```python
from build123d import *

# Parameters (mm, degrees)
SKETCH1_W                = 304.8
SKETCH1_H                = 304.8
BOSS_EXTRUDE1_DEPTH      = 2.54
SKETCH2_W                = 64.109804122
SKETCH2_H                = 40.213084064
BOSS_EXTRUDE2_DEPTH      = 31.75
BOSS_EXTRUDE2_TAPER      = 6
SKETCH3_R                = 6.35
CUT_EXTRUDE1_DEPTH       = 25.4
BOSS_EXTRUDE3_DEPTH      = 19.05
BOSS_EXTRUDE3_DEPTH_BACK = 19.05
SKETCH5_R                = 6.35
CUT_EXTRUDE2_DEPTH       = 50.8
SKETCH6_R                = 6.35
CUT_EXTRUDE3_DEPTH       = 19.05


with BuildPart() as part:
    # Sketch1 → Boss-Extrude1 (new body)
    with BuildSketch(Plane(origin=(0, 0, 0), x_dir=(1, 0, 0), z_dir=(0, 1, 0))):
        with Locations((152.4, 152.4)):
            Rectangle(SKETCH1_W, SKETCH1_H)
    extrude(amount=BOSS_EXTRUDE1_DEPTH)

    # Sketch2 → Boss-Extrude2 (add)
    with BuildSketch(Plane(origin=(0, 2.54, 0), x_dir=(1, 0, 0), z_dir=(0, 1, 0))):
        with Locations((152.4, 228.6)):
            Rectangle(SKETCH2_W, SKETCH2_H)
    extrude(amount=BOSS_EXTRUDE2_DEPTH, taper=BOSS_EXTRUDE2_TAPER)

    # Sketch3 → Cut-Extrude1 (cut)
    with BuildSketch(Plane(origin=(0, 34.29, 0), x_dir=(1, 0, 0), z_dir=(0, 1, 0))):
        with Locations((152.4, 228.6)):
            Circle(SKETCH3_R)
    extrude(amount=-CUT_EXTRUDE1_DEPTH, mode=Mode.SUBTRACT)

    # Sketch4 → Boss-Extrude3 (add, two sides)
    with BuildSketch(Plane(origin=(152.4, 0, 0), x_dir=(0, 0, -1), z_dir=(1, 0, 0))) as boss_extrude3_sk:
        Polygon((209.648741009, 34.29), (247.551258991, 34.29), (247.551258991, 36.83), (212.188741009, 36.83), (212.188741009, 77.47), (212.188741009, 85.09), (209.648741009, 85.09), align=None)
    extrude(amount=BOSS_EXTRUDE3_DEPTH)
    extrude(boss_extrude3_sk.sketch, amount=-BOSS_EXTRUDE3_DEPTH_BACK)

    # Sketch5 → Cut-Extrude2 (cut)
    with BuildSketch(Plane(origin=(0, 36.83, 0), x_dir=(1, 0, 0), z_dir=(0, 1, 0))):
        with Locations((152.4, 228.6)):
            Circle(SKETCH5_R)
    extrude(amount=-CUT_EXTRUDE2_DEPTH, mode=Mode.SUBTRACT)

    # Sketch6 → Cut-Extrude3 (cut)
    with BuildSketch(Plane(origin=(0, 0, -212.188741009), x_dir=(-1, 0, 0), z_dir=(0, 0, -1))):
        with Locations((-152.4, 71.864665845)):
            Circle(SKETCH6_R)
        with Locations((-152.4, 51.544665845)):
            Circle(SKETCH6_R)
    extrude(amount=-CUT_EXTRUDE3_DEPTH, mode=Mode.SUBTRACT)


solid = part.part
```
Design review of the part built by this model. Coordinates are the model's own, in mm. A direction names the side the tool comes from. Give positions to 0.01 mm unless a question says otherwise; leave off trailing zeros. Order: outer loops, then holes, each group sorted by start corner. A loop starts at its lowest first (then second) coordinate and runs counter-clockwise, first axis right, second up. Notation, with made-up numbers: (-12, 16) -> (37, 16) arc R14 cw to (37, 21) -> close; hole circle Ø9 at (-26.75, 9.25). An arc over 180 degrees is marked (long way). Write item = value, one per line. Start each with the question number.
(1) Mouldability with a two-part tool opening along X and no side actions: class faces 5 (the face through (133.35, 52, -212)), 6 (the face through (151.02, 18.67, -222.4)), 7 (the face through (153, 60, -209.649)) as +X half, -X half, draft (parallel to the pull), parting line (faces both ways), or undercut.
(2) We need section B-B on z = -44. Write out the cut boundary in (x, y).
(3) To check wall thickness, follow line 1 along Z through (x, y) = (152, 13); line 2 along Y through (x, z) = (63, -51); line 3 along Y through (x, z) = (177, -236). State the ranges of each line that lie inside material, in increasing order.
(4) For pin 1 (11.5 mm diameter, centred on x = 152.4, y = 51.54, fed in from +Z); pin 2 (16.5 mm diameter, centred on x = 152.4, y = 71.86, fed in from -Z); pin 3 (2.5 mm diameter, centred on x = 155.5, z = -211.5, fed in from -Y); pin 4 (17.5 mm diameter, centred on x = 157, z = -238, fed in from +Y), all flat-tipped, find the tip position at first contact; note any pin that passes through.
(5) For faces 1 (the face through (146.534, 69.433, -210.937)), 2 (the face through (128, 34.29, -229)), 3 (the face through (176, 34.29, -229)), 4 (the face through (157, 36.83, -234)), list the 3-axis set-ups (+Z, -Z, +X, -X, +Y, -Y) from which the entire face can be reached by the end or side of a thin tool; tool diameter is ignored.
(6) We need section C-C on x = 100.5. Write out the cut boundary in (y, z).
(7) We need section A-A on x = 152.4. State how many separate pieces and enclosed holes the cut face has, plus the area to 3 significant figures.
Numbers:
q1.face_5 = -X half
q1.face_6 = undercut
q1.face_7 = draft
q2.outline = (0, 0) -> (304.8, 0) -> (304.8, 2.54) -> (0, 2.54) -> close
q3.line_1 = -247.61 to -234.94, -222.26 to -209.59
q3.line_2 = 0 to 2.54
q3.line_3 = 0 to 34.29
q4.pin_1 = through
q4.pin_2 = -212.19
q4.pin_3 = 0
q4.pin_4 = 36.83
q5.face_1 = +Z, -Z
q5.face_2 = +Z, -Z, -X, +Y
q5.face_3 = +Z, -Z, +X, +Y
q5.face_4 = -Z, +X, -X, +Y
q6.outline = (0, -304.8) -> (2.54, -304.8) -> (2.54, 0) -> (0, 0) -> close
q7.separate_pieces = 4
q7.enclosed_holes = 0
q7.area = 1,630 mm^2
